The listing builds one solid part. Answer for the finished solid, in the listing's coordinates (mm). Coordinates: 2 decimals unless noted, no trailing zeros. Order: outer loops, then holes, each group sorted by start corner. A loop starts at its lowest first (then second) coordinate and runs counter-clockwise, first axis right, second up. Notation, with made-up numbers: (47.5, 55.5) -> (53.5, 55.5) arc R29 ccw to (53.5, 76.5) -> close; hole circle Ø5 at (19, 56). An arc over 180 degrees is marked (long way). Write item = value, one per line.
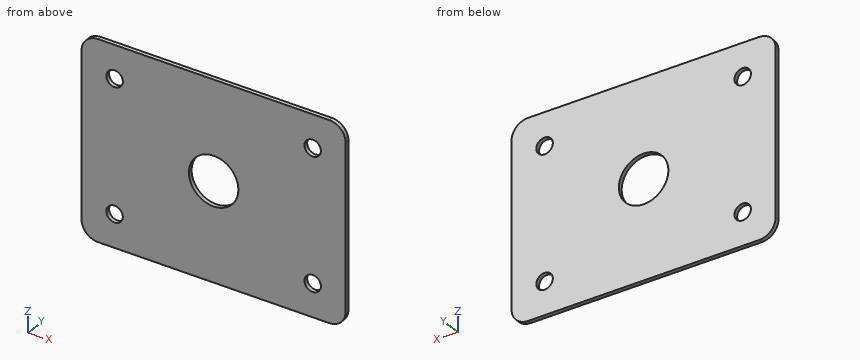
from build123d import *

# Parameters (mm, degrees)
F0_W     = 101.6
F0_H     = 76.2
F0_R     = 3.175
F0_R_2   = 9.525
F1_DEPTH = 1.5875
F2_R     = 6.35


with BuildPart() as f1:
    # F0 (on Front) → F1 (new body)
    with BuildSketch(Plane.XZ):
        Rectangle(F0_W, F0_H)
        with Locations((-38.1, -25.4)):
            Circle(F0_R, mode=Mode.SUBTRACT)
        with Locations((38.1, -25.4)):
            Circle(F0_R, mode=Mode.SUBTRACT)
        Circle(F0_R_2, mode=Mode.SUBTRACT)
        with Locations((-38.1, 25.4)):
            Circle(F0_R, mode=Mode.SUBTRACT)
        with Locations((38.1, 25.4)):
            Circle(F0_R, mode=Mode.SUBTRACT)
    extrude(amount=F1_DEPTH)

    # F2
    f2_edges = [f1.edges().sort_by_distance(p)[0] for p in [
        (50.8, -0.79375, 38.1),
        (50.8, -0.79375, -38.1),
        (-50.8, -0.79375, -38.1),
        (-50.8, -0.79375, 38.1),
    ]]
    fillet(f2_edges, radius=F2_R)


solid = f1.part
Q1. Section B-B, the plane z = 25.4 is taken. Give the vertices of the cut face in (x, y) (1 decimal).
The answers:
outline = (-50.8, -1.6) -> (-41.3, -1.6) -> (-41.3, 0) -> (-50.8, 0) -> close; (-34.9, -1.6) -> (34.9, -1.6) -> (34.9, 0) -> (-34.9, 0) -> close; (41.3, -1.6) -> (50.8, -1.6) -> (50.8, 0) -> (41.3, 0) -> close
Q2. Section A-A, the plane x = 0 is taken. Give the vertices of the cut face in (y, z) (1 decimal), plus the area to 3 significant figures.
The answers:
outline = (-1.6, -38.1) -> (0, -38.1) -> (0, -9.5) -> (-1.6, -9.5) -> close; (-1.6, 9.5) -> (0, 9.5) -> (0, 38.1) -> (-1.6, 38.1) -> close
area = 90.7 mm2
Q3. Section C-C, the plane x = -38.1 is taken. Give the vertices of the cut face in (y, z) (1 decimal), plus the area to 3 significant figures.
The answers:
outline = (-1.6, -38.1) -> (0, -38.1) -> (0, -28.6) -> (-1.6, -28.6) -> close; (-1.6, -22.2) -> (0, -22.2) -> (0, 22.2) -> (-1.6, 22.2) -> close; (-1.6, 28.6) -> (0, 28.6) -> (0, 38.1) -> (-1.6, 38.1) -> close
area = 101 mm2
Q4. This flat-tipped pin is pushed along its axis until it touches: pin 1 Ø8 at (x, z) = (5.5, 25) entering from +Y. Where does it stop, or does it pass through?
The answers:
pin_1 = 0
Q5. Find the intervals of material crossed by line 1 along X through (y, z) = (-1.2, -25); line 2 along Z through (x, y) = (-38.1, -0.5) (3 decimals); line 3 along Z through (x, y) = (-36, -0.55), in increasing order.
The answers:
line_1 = -50.8 to -41.25, -34.95 to 34.95, 41.25 to 50.8
line_2 = -38.1 to -28.575, -22.225 to 22.225, 28.575 to 38.1
line_3 = -38.1 to -27.78, -23.02 to 23.02, 27.78 to 38.1
Q6. Section D-D, the plane y = -0.35 is taken. Give the vertices of the cut face in (x, z) (3 decimals).
The answers:
outline = (-50.8, -31.75) arc R6.35 ccw to (-44.45, -38.1) -> (44.45, -38.1) arc R6.35 ccw to (50.8, -31.75) -> (50.8, 31.75) arc R6.35 ccw to (44.45, 38.1) -> (-44.45, 38.1) arc R6.35 ccw to (-50.8, 31.75) -> close; hole circle Ø6.35 at (-38.1, -25.4); hole circle Ø6.35 at (-38.1, 25.4); hole circle Ø19.05 at (0, 0); hole circle Ø6.35 at (38.1, -25.4); hole circle Ø6.35 at (38.1, 25.4)
